```python
from build123d import *

# Parameters (mm, degrees)
F0_R     = 6.5898328627
F1_DEPTH = 12.7
F3_DEPTH = 6.35
F4_SIZE  = 1.016
F6_D     = 6.35


with BuildPart() as f1:
    # F0 (on Front) → F1 (new body)
    with BuildSketch(Plane.XZ):
        with BuildLine():
            Line((5.9883656788, 26.1059254408), (-45.6207543612, 26.1059254408))
            Line((-45.6207543612, 26.1059254408), (-45.6207543612, 2.8432162944))
            Line((-45.6207543612, 2.8432162944), (46.3961809874, 2.8432162944))
            Line((46.3961809874, 2.8432162944), (46.3961809874, 26.1059254408))
            Line((46.3961809874, 26.1059254408), (26.3209578705, 26.1059254408))
            ThreePointArc((26.3209578705, 26.1059254408), (27.9321742637, 22.7805506138), (28.4858180464, 19.127111882))
            ThreePointArc((28.4858180464, 19.127111882), (12.5012230428, 7.3495993929), (5.9883656788, 26.1059254408))
        make_face()
        with Locations((-31.9216027856, 16.5423676372)):
            Circle(F0_R, mode=Mode.SUBTRACT)
        with BuildLine():
            ThreePointArc((26.3209578705, 26.1059254408), (16.1546617746, 31.4582681537), (5.9883656788, 26.1059254408))
            Line((5.9883656788, 26.1059254408), (26.3209578705, 26.1059254408))
        make_face()
        with BuildLine():
            Line((26.3209578705, 26.1059254408), (5.9883656788, 26.1059254408))
            ThreePointArc((5.9883656788, 26.1059254408), (12.5012230428, 7.3495993929), (28.4858180464, 19.127111882))
            ThreePointArc((28.4858180464, 19.127111882), (27.9321742637, 22.7805506138), (26.3209578705, 26.1059254408))
        make_face()
    extrude(amount=F1_DEPTH)

    # F2 (on face) → F3 (join)
    with BuildSketch(Plane(origin=(0, 0, 0), x_dir=(-1, 0, 0), z_dir=(0, 1, 0))):
        Polygon((6.7886244506, 26.1059254408), (4.4478680938, 2.8432162944), (8.4228813648, 2.8432162944), (10.5955973268, 26.1059254408), align=None)
    extrude(amount=F3_DEPTH)

    # F4
    f4_edges = [f1.edges().sort_by_distance(p)[0] for p in [
        (-9.509239, 6.35, 14.474571),
        (-5.618246, 6.35, 14.474571),
        (20.974156, 0, 2.843216),
        (-27.021818, 0, 2.843216),
        (-38.511436, 0, 16.542368),
        (16.154662, 0, 31.458268),
        (-0.400129, 0, 26.105925),
        (-28.108176, 0, 26.105925),
        (-45.620754, 0, 14.474571),
        (46.396181, 0, 14.474571),
        (36.358569, 0, 26.105925),
    ]]
    chamfer(f4_edges, length=F4_SIZE)

    # F6 (through all)
    with Locations(Plane(origin=(0, 0, 0), x_dir=(-1, 0, 0), z_dir=(0, 1, 0))):
        with Locations((-16.4722520858, 23.0548288673)):
            Hole(F6_D / 2)


solid = f1.part
```
The listing builds one solid part. Answer for the finished solid, in the listing's coordinates (mm). A direction names the side the tool comes from. Coordinates: 2 decimals unless noted, no trailing zeros. Loops run counter-clockwise (first coordinate to the right, second up) from the corner with the lowest first, then second, coordinate; pieces in that order, holes last. Notation, with made-up numbers: (60.25, -37) -> (80.25, -37) arc R19 cw to (80.25, -29) -> close; hole circle Ø4 at (3.25, 42.25). An arc over 180 degrees is marked (long way). Return JSON: item names as keys, results as strings. Group by question number.
(1) Determine the mould class of faces 3 (the cylindrical face through (14.13, -6.44, 25.2)), 4 (the flat face through (36, -7, 26.106)), 5 (the cylindrical face through (16.322, -6.776, 31.457)), 6 (the cylindrical face through (-38.505, -6.776, 16.832)) for opening direction X: released by +X, released by -X, zero draft, split by the parting line, or undercut.
(2) A cutting plane is placed at A-A on x = -21.5. Write down the section's boundary in (y, z).
(3) Given pin 1 Ø5 at (x, z) = (14, 8.5) entering from +Y; pin 2 Ø9.5 at (x, y) = (36.5, -9) entering from +Z, each flat-ended and moving along its own axis, determine where each tip first touches the part or whether it passes through.
(4) Which of the six approach directions +Z, -Z, +X, -X, +Y, -Y give full straight-line access (tool end or side, diameter ignored) to faces 1 (the flat face through (-19, -7, 26.106)), 2 (the flat face through (46.396, -7, 14))?
(5) A cutting plane is placed at C-C on z = 6.75. Write down the section's boundary in (x, y).
(6) Find the intervals of material crossed by probe 1 along Z at (x, y) = (-11, -7.25); probe 2 along X at (y, z) = (-12, 23.25); probe 3 along Y at (x, z) = (26.5, 20), in increasing order. Write a range as from..to.
(7) A cutting plane is placed at B-B on y = -4.25. Write down the section's boundary in (x, z) (3 decimals), and give its area (3 significant figures).
(8) A cutting plane is placed at D-D on y = 1. Write down the section's boundary in (x, z).
The answers:
{
 "1": {"face 3": "undercut", "face 4": "zero draft", "face 5": "split by the parting line", "face 6": "undercut"},
 "2": {"outline": "(-12.7, 2.84) -> (-1.02, 2.84) -> (0, 3.86) -> (0, 25.09) -> (-1.02, 26.11) -> (-12.7, 26.11) -> close"},
 "3": {"pin 1": "stops at y = 0", "pin 2": "stops at z = 26.11"},
 "4": {"face 1": "+Z, -X, +Y, -Y", "face 2": "+Z, -Z, +X, +Y, -Y"},
 "5": {"outline": "(-45.62, -12.7) -> (46.4, -12.7) -> (46.4, -1.02) -> (45.38, 0) -> (-4.84, 0) -> (-4.84, 5.33) -> (-5.86, 6.35) -> (-7.77, 6.35) -> (-8.79, 5.33) -> (-8.79, 0) -> (-44.6, 0) -> (-45.62, -1.02) -> close"},
 "6": {"probe 1": "z = 2.84..26.11", "probe 2": "x = -45.62..13.3, 19.64..46.4", "probe 3": "y = -12.7..0"},
 "7": {"outline": "(-45.621, 2.843) -> (46.396, 2.843) -> (46.396, 26.106) -> (26.321, 26.106) arc R12.331 ccw to (5.988, 26.106) -> (-45.621, 26.106) -> close; hole circle Ø13.18 at (-31.922, 16.542); hole circle Ø6.35 at (16.472, 23.055)", "area": "2,050 mm^2"},
 "8": {"outline": "(-10.6, 26.11) -> (-8.42, 2.84) -> (-4.45, 2.84) -> (-6.79, 26.11) -> close"}
}
